Read the model definition and answer for the solid it produces. Units are mm, in the model's axes. Coordinates: 2 decimals unless noted, no trailing zeros. Order: outer loops, then holes, each group sorted by start corner. A loop starts at its lowest first (then second) coordinate and runs counter-clockwise, first axis right, second up. Notation, with made-up numbers: (-31, 87) -> (-25, 87) arc R14 ccw to (-25, 113) -> close; hole circle Ø11 at (89, 40). An arc over 180 degrees is marked (long way). Return JSON: item names as keys, results as strings. Group by question number.
```python
from build123d import *

# Parameters (mm, degrees)
F1_DEPTH = 6.35


with BuildPart() as f1:
    # F0 (on Top) → F1 (new body)
    with BuildSketch(Plane.XY):
        Polygon((-79.022222, 95.25), (-79.022222, 101.6), (-101.6, 101.6), (-101.6, 79.022222), (-95.25, 79.022222), (-95.25, 56.444444), (-101.6, 56.444444), (-101.6, 33.866667), (-95.25, 33.866667), (-95.25, 11.288889), (-101.6, 11.288889), (-101.6, 0), (-101.6, -11.288889), (-95.25, -11.288889), (-95.25, -33.866667), (-101.6, -33.866667), (-101.6, -56.444444), (-95.25, -56.444444), (-95.25, -79.022222), (-101.6, -79.022222), (-101.6, -101.6), (-79.022222, -101.6), (-79.022222, -95.25), (-56.444444, -95.25), (-56.444444, -101.6), (-33.866667, -101.6), (-33.866667, -95.25), (-11.288889, -95.25), (-11.288889, -101.6), (11.288889, -101.6), (11.288889, -95.25), (33.866667, -95.25), (33.866667, -101.6), (56.444444, -101.6), (56.444444, -95.25), (79.022222, -95.25), (79.022222, -101.6), (95.25, -101.6), (95.25, -79.022222), (101.6, -79.022222), (101.6, -56.444444), (95.25, -56.444444), (95.25, -33.866667), (101.6, -33.866667), (101.6, -11.288889), (95.25, -11.288889), (95.25, 0), (95.25, 11.288889), (101.6, 11.288889), (101.6, 33.866667), (95.25, 33.866667), (95.25, 56.444444), (101.6, 56.444444), (101.6, 79.022222), (95.25, 79.022222), (95.25, 101.6), (79.022222, 101.6), (79.022222, 95.25), (56.444444, 95.25), (56.444444, 101.6), (33.866667, 101.6), (33.866667, 95.25), (11.288889, 95.25), (11.288889, 101.6), (-11.288889, 101.6), (-11.288889, 95.25), (-33.866667, 95.25), (-33.866667, 101.6), (-56.444444, 101.6), (-56.444444, 95.25), align=None)
    extrude(amount=F1_DEPTH)


solid = f1.part
```
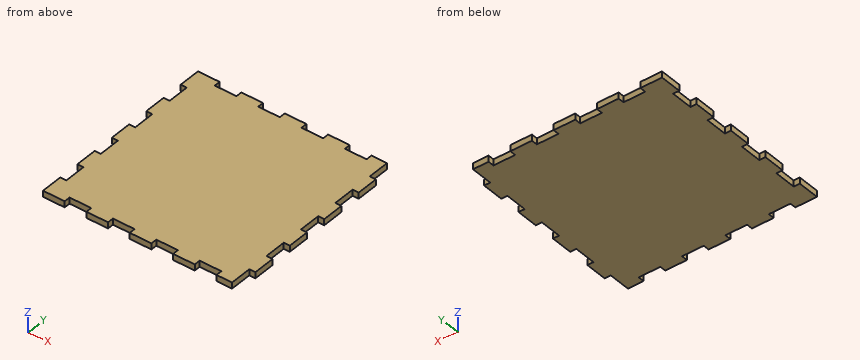
1. Given pin 1 (3 mm diameter, centred on x = 69, z = 1, fed in from +Y); pin 2 (3 mm diameter, centred on x = 98, z = 3, fed in from +Y); pin 3 (1 mm diameter, centred on x = -24.5, z = 5, fed in from -Y), each flat-ended and moving along its own axis, determine where each tip first touches the part or whether it passes through.
2. Straight lines are drawn through the part: L1, parallel to Y at x = -32.5, z = 5.25; L2, parallel to X at y = 9.5, z = 4.75; L3, parallel to X at y = 57, z = 2. For each, find the intervals that lie inside material, in ascending order.
3. Find section B-B on y = -69. Determine the outline of the cut face in (x, z), and give its area (3 significant figures).
4. Find section A-A on x = -26. Determine the outline of the cut face in (y, z).
Result:
{
 "1": {"pin 1": "y = 95.25", "pin 2": "y = 79.02", "pin 3": "y = -95.25"},
 "2": {"L1": "-95.25 to 95.25", "L2": "-101.6 to 95.25", "L3": "-95.25 to 101.6"},
 "3": {"outline": "(-95.25, 0) -> (101.6, 0) -> (101.6, 6.35) -> (-95.25, 6.35) -> close", "area": "1,250 mm^2"},
 "4": {"outline": "(-95.25, 0) -> (95.25, 0) -> (95.25, 6.35) -> (-95.25, 6.35) -> close"}
}
